Can you work these out from the model? Positions are in its coordinate system, mm. A direction names the side the tool comes from. Round coordinates to 2 decimals unless told otherwise and drop trailing zeros. Write each loop counter-clockwise with the first axis right and the second up, starting at its lowest first coordinate (ties: lowest second). Pieces come first, ordered by that corner, then holes.
Q1. For faces 4 (the flat face through (41, -18.6, -5)), 5 (the flat face through (18.6, 0, -5)), 6 (the flat face through (-19.66, 0.29, -3.09)), 7 (the flat face through (48.501, 0.266, 11.437)), which set-ups out of +Z, -Z, +X, -X, +Y, -Y let a thin tool reach every point of the face, with its end or its side?
Q2. If we section it at B-B (x = 56.5): Please give me the cut outline in (y, z).
Q3. I'm going to push flat-ended pins straight in: pin 1 Ø0.5 at (x, z) = (34, -5.5) entering from -Y; pin 2 Ø1.4 at (y, z) = (-4, -5) entering from -X; pin 3 Ø1.4 at (x, z) = (41.5, -5) entering from +Y; pin 4 Ø12 at (x, y) = (-9.5, -4.5) entering from +Z. Where does each tip first touch, or does it pass through?
Q4. If we section it at C-C (y = -16): Please give me the cut outline in (x, z), plus the area to 3 significant figures.
Q5. Please list where these lines run through material, in increasing order: line 1 along Z through (x, y) = (7, -0.5); line 2 along Y through (x, z) = (16.5, 14.25); line 3 along X through (y, z) = (8, 13.25).
Q6. We'd pull the mould along Y, two halves only. Please class faces 1 (the flat face through (20, 20.75, 7)), 2 (the flat face through (19, 7.762, 11)), 3 (the flat face through (62.25, 0, 7)): +Y half, -Y half, draft (parallel to the pull), parting line (faces both ways), or undercut.
Q7. If we section it at D-D (y = 1.5): Please give me the cut outline in (x, z).
Autodesk Fusion 360 part; units mm, degrees
sketch "Sketch1" plane through (0, 0, 0) normal (0, 0, 1) x (1, 0, 0)
  line L0 (20.75, 20.75) -> (-20.75, 20.75)
  line L1 (-20.75, 20.75) -> (-20.75, -20.75)
  line L2 (-20.75, -20.75) -> (20.75, -20.75)
  line L3 (20.75, -20.75) -> (20.75, 20.75)
  line L4 (20.75, 20.75) -> (-20.75, -20.75) construction
  line L5 (-20.75, 20.75) -> (20.75, -20.75) construction
  dimension "d1" = 41.5
  dimension "d2" = 41.5
extrude "Extrude1" add sketch "Sketch1" along normal blind 7 makes body 1
sketch "Sketch2" plane through (0, 20.75, 0) normal (0, 1, 0) x (-1, 0, 0)
  line L0 (-20.75, 0) -> (20.75, 0)
  line L1 (20.75, 0) -> (20.75, 7)
  line L2 (20.75, 7) -> (-20.75, 7)
  line L3 (-20.75, 7) -> (-20.75, 0)
  line L4 (18.6, 0.8) -> (18.6, 2.6)
  line L5 (18.6, 2.6) -> (20.75, 4.75)
  line L6 (17.8, 0) -> (18.6, 0.8)
  line L7 (-18.6, 0.9534) -> (-18.6, 2.7534)
  line L8 (-18.6, 2.7534) -> (-20.75, 4.9034)
  line L9 (-17.8, 0) -> (-18.6, 0.9534)
  line L10 (-20.75, 4.9034) -> (-20.75, 0)
  line L11 (-20.75, 0) -> (-17.8, 0)
  line L12 (20.75, 4.75) -> (20.75, 0)
  line L13 (17.8, 0) -> (20.75, 0)
sketch "Sketch3" plane through (-20.75, 0, 0) normal (-1, 0, 0) x (0, -1, 0)
  line L0 (20.75, 7) -> (-20.75, 7)
  line L1 (-20.75, 0) -> (-17.8, 0)
  line L2 (-17.8, 0) -> (-18.6, 0)
  line L3 (-17.8, 0) -> (-18.6, 0.8)
  line L4 (-17.8, 0) -> (-12.38, 0) construction
  line L5 (-18.6, 0.8) -> (-18.6, 2.6)
  line L6 (-18.6, 2.6) -> (-20.75, 4.75)
  line L7 (17.8, 0) -> (18.6, 0.8)
  line L8 (18.6, 0.8) -> (18.6, 2.6)
  line L9 (18.6, 2.6) -> (20.75, 4.75)
  line L10 (20.75, 4.75) -> (20.75, 0)
  line L11 (20.75, 0) -> (17.8, 0)
  line L12 (-20.75, 4.75) -> (-20.75, 0)
sketch "Sketch4" plane through (0, -20.75, 0) normal (0, -1, 0) x (1, 0, 0)
  line L0 (-20.75, 0) -> (20.75, 0)
  line L1 (20.75, 0) -> (20.75, 7)
  line L2 (20.75, 7) -> (-20.75, 7)
  line L3 (-20.75, 7) -> (-20.75, 0)
  line L4 (-20.75, 0) -> (-17.8, 0)
  line L5 (-17.8, 0) -> (-18.6, 0)
  line L6 (-17.8, 0) -> (-18.6, 0.8)
  line L7 (-17.8, 0) -> (-12.5744, 0) construction
  line L8 (-18.6, 0.8) -> (-18.6, 2.6)
  line L9 (-18.6, 2.6) -> (-20.75, 4.75)
  line L10 (20.75, 0) -> (17.8, 0)
  line L11 (17.8, 0) -> (18.6, 0)
  line L12 (17.8, 0) -> (18.6, 0.8)
  line L13 (18.6, 0.8) -> (18.6, 2.6)
  line L14 (18.6, 2.6) -> (20.75, 4.75)
sketch "Sketch5" plane through (20.75, 0, 0) normal (1, 0, 0) x (0, 1, 0)
  line L0 (-20.75, 0) -> (20.75, 0)
  line L1 (20.75, 0) -> (20.75, 7)
  line L2 (20.75, 7) -> (-20.75, 7)
  line L3 (-20.75, 7) -> (-20.75, 0)
  line L4 (-20.75, 0) -> (-17.8, 0)
  line L5 (-17.8, 0) -> (-18.6, 0)
  line L6 (-17.8, 0) -> (-18.6, 0.8)
  line L7 (-18.6, 0.8) -> (-18.6, 2.6)
  line L8 (-18.6, 2.6) -> (-20.75, 4.75)
  line L9 (20.75, 0) -> (17.8, 0)
  line L10 (17.8, 0) -> (18.6, 0)
  line L11 (18.6, 0.8) -> (18.6, 2.6)
  line L12 (18.6, 2.6) -> (20.75, 4.75)
  line L13 (17.8, 0) -> (18.6, 0.8)
extrude "Extrude2" cut sketch "Sketch5" along normal mid plane 100 contours L0 L3 L4 L5 L6 L7 L8 | L0 L1 L9 L10 L11 L12 L13 bodies 1
extrude "Extrude3" cut sketch "Sketch4" along normal mid plane 100 contours L0 L3 L4 L5 L6 L8 L9 | L0 L1 L10 L11 L12 L13 L14 bodies 1
copy_body "CopyPasteBodies1" bodies 1 makes body 2
move_body "Move1" bodies 2 to x (1, 0, 0) y (0, 1, 0) z (0, 0, 1) at (41.5, 0, 0)
combine "Combine1" operation add target body 1 tool bodies 2
sketch "Sketch6" plane through (0, 0, 7) normal (0, 0, 1) x (-1, 0, 0)
  line L0 (-62.25, -20.75) -> (20.75, -20.75)
  line L1 (20.75, -20.75) -> (20.75, 20.75)
  line L2 (20.75, 20.75) -> (-62.25, 20.75)
  line L3 (-62.25, 20.75) -> (-62.25, -20.75)
  line L4 (10.0352, -4.2687) -> (6.3028, -4.1922)
  line L5 (6.3028, -4.1922) -> (6.0326, -11.9325)
  line L6 (6.0326, -11.9325) -> (-17.7748, -11.649)
  line L7 (-17.7748, -11.649) -> (-17.7285, -7.7618)
  line L8 (-17.7285, -7.7618) -> (-20.7225, -7.7618)
  line L9 (-20.7225, -7.7618) -> (-20.7225, -2.3106)
  line L10 (-20.7225, -2.3106) -> (-45.8884, -2.3106)
  line L11 (-45.8884, -2.3106) -> (-51.1886, 1.836)
  line L12 (-51.1886, 1.836) -> (-46.6533, 7.6332)
  line L13 (-46.6533, 7.6332) -> (-20.3871, 7.0947)
  line L14 (-20.3871, 7.0947) -> (-20.2261, 14.9498)
  line L15 (-20.2261, 14.9498) -> (8.0521, 14.37)
  line L16 (8.0521, 14.37) -> (7.8807, 6.0104)
  line L17 (7.8807, 6.0104) -> (10.245, 5.9619)
  line L18 (10.245, 5.9619) -> (10.0352, -4.2687)
sketch "Sketch7" plane through (0, 0, 0) normal (0, 0, 1) x (1, 0, 0)
  line L0 (-20.75, 20.75) -> (62.25, 20.75)
  line L1 (62.25, 20.75) -> (62.25, -20.75)
  line L2 (62.25, -20.75) -> (-20.75, -20.75)
  line L3 (-20.75, -20.75) -> (-20.75, 20.75)
move_body "Move2" bodies 1 to x (1, 0, 0) y (0, 1, 0) z (0, 0, 1) at (0, 0, -6.75)
extrude "Extrude4" add sketch "Sketch7" along normal blind 16 separate body makes body 3
combine "Combine2" operation add target body 3 tool bodies 1
extrude "Extrude5" cut sketch "Sketch6" along normal blind 16 contours L4 L5 L6 L7 L8 L9 L10 L11 L12 L13 L14 L15 L16 L17 L18 bodies 3
A:
1. face 4: -Z, +X, -X, -Y
1. face 5: -Z, +Y, -Y
1. face 6: -Z, -X, +Y, -Y
1. face 7: +Z
2. outline: (-20.75, -2) - (-18.6, -4.15) - (-18.6, -5.95) - (-17.8, -6.75) - (17.8, -6.75) - (18.6, -5.95) - (18.6, -4.15) - (20.75, -2) - (20.75, 16) - (-20.75, 16) - close
3. pin 1: stops at y = -18.6
3. pin 2: stops at x = -18.6
3. pin 3: stops at y = 18.6
3. pin 4: stops at z = 16
4. outline: (-20.75, -2) - (-18.6, -4.15) - (-18.6, -5.95) - (-17.8, -6.75) - (17.8, -6.75) - (18.6, -5.95) - (18.6, -4.15) - (20.75, -2) - (22.9, -4.15) - (22.9, -5.95) - (23.7, -6.75) - (59.3, -6.75) - (60.1, -5.95) - (60.1, -4.15) - (62.25, -2) - (62.25, 16) - (-20.75, 16) - close
4. area: 1,860 mm2
5. line 1: z = -6.75 to 7
5. line 2: y = -20.75 to -14.87, 11.66 to 20.75
5. line 3: x = -20.75 to -6.17, 17.73 to 62.25
6. face 1: +Y half
6. face 2: undercut
6. face 3: draft
7. outline: (-20.75, -2) - (-18.6, -4.15) - (-18.6, -5.95) - (-17.8, -6.75) - (17.8, -6.75) - (18.6, -5.95) - (18.6, -4.15) - (20.75, -2) - (22.9, -4.15) - (22.9, -5.95) - (23.7, -6.75) - (59.3, -6.75) - (60.1, -5.95) - (60.1, -4.15) - (62.25, -2) - (62.25, 16) - (46.92, 16) - (46.92, 7) - (-10.09, 7) - (-10.09, 16) - (-20.75, 16) - close
